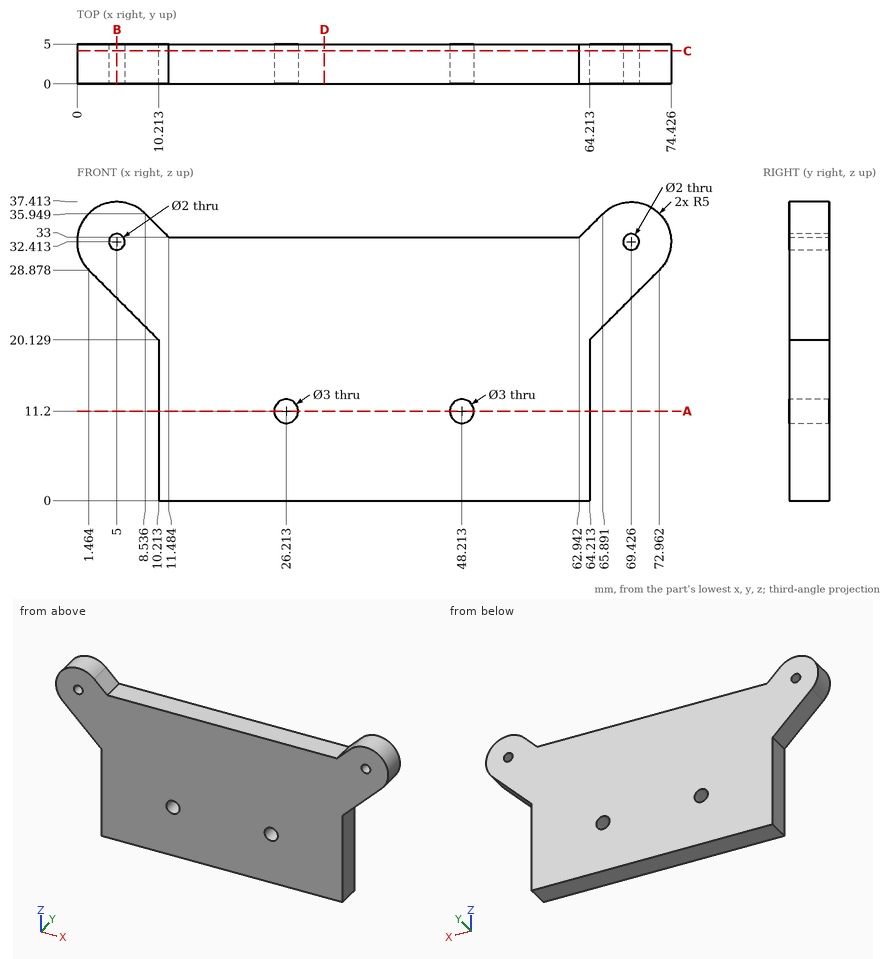
Here's the drawing with two shaded views (mm, measured from the low corner). I have some questions. Give positions to 0.01 mm unless a question says otherwise; leave off trailing zeros. Write each loop counter-clockwise with the first axis right and the second up, starting at its lowest first coordinate (ties: lowest second). Pieces come first, ordered by that corner, then holes. Notation, with made-up numbers: (21.5, 86) - (74.5, 86) arc R18 ccw to (74.5, 99) - close; hole circle Ø2 at (85, 6.25). An arc over 180 degrees is marked (long way). Write item = value, one per line. Start each with the question number.
1. Imagine slicing it at A-A (z = 11.2). Please give me the cut outline in (x, y), and give its area (3 significant figures).
2. Imagine slicing it at C-C (y = 4.15). Please give me the cut outline in (x, z) (1 decimal).
3. Imagine slicing it at D-D (x = 31). Please give me the cut outline in (y, z), and give its area (3 significant figures).
4. Please list where these lines run through material, in increasing order: line 1 (X direction, y = 3.4, z = 11.2); line 2 (X direction, y = 1.9, z = 13.5); line 3 (Z direction, x = 34.5, y = 2.35).
5. For pin 1 (3 mm diameter, centred on x = 38.5, y = 2.5, fed in from +Z); pin 2 (1.5 mm diameter, centred on y = 2, z = 7, fed in from +X), each with a flat end and sliding along its axis, tell me the tip position at first contact or that it passes through.
6. Imagine slicing it at B-B (x = 5). Please give me the cut outline in (y, z).
Worked answers:
q1.outline = (10.21, 0) - (24.71, 0) - (24.71, 5) - (10.21, 5) - close; (27.71, 0) - (46.71, 0) - (46.71, 5) - (27.71, 5) - close; (49.71, 0) - (64.21, 0) - (64.21, 5) - (49.71, 5) - close
q1.area = 240 mm2
q2.outline = (1.5, 28.9) - (10.2, 20.1) - (10.2, 0) - (64.2, 0) - (64.2, 20.1) - (73, 28.9) arc R5 ccw to (65.9, 35.9) - (62.9, 33) - (11.5, 33) - (8.5, 35.9) arc R5 ccw to start; hole circle Ø2 at (5, 32.4); hole circle Ø3 at (26.2, 11.2); hole circle Ø3 at (48.2, 11.2); hole circle Ø2 at (69.4, 32.4)
q3.outline = (0, 0) - (5, 0) - (5, 33) - (0, 33) - close
q3.area = 165 mm2
q4.line_1 = 10.21 to 24.71, 27.71 to 46.71, 49.71 to 64.21
q4.line_2 = 10.21 to 64.21
q4.line_3 = 0 to 33
q5.pin_1 = 33
q5.pin_2 = 64.21
q6.outline = (0, 25.34) - (5, 25.34) - (5, 31.41) - (0, 31.41) - close; (0, 33.41) - (5, 33.41) - (5, 37.41) - (0, 37.41) - close
